Geometry check sheet. Reference: the model listing, model coordinates, mm. A direction names the side the tool comes from. Give positions to 0.01 mm unless a question says otherwise; leave off trailing zeros. Write each loop counter-clockwise with the first axis right and the second up, starting at its lowest first coordinate (ties: lowest second). Pieces come first, ordered by that corner, then holes.
(1) Tool access check on faces 4 (the flat face through (0, -1.588, -118)), 5 (the cylindrical face through (0.488, -0.805, -185.804)). Record the directions out of +Z, -Z, +X, -X, +Y, -Y that give a thin tool (end or side, any length) a straight path to the whole face; none if there is none.
(2) Cross-section at C-C (z = -180). Record the boundary of the cut face in (x, y).
(3) Cross-section at A-A (y = -9). Record the boundary of the cut face in (x, z).
(4) Cross-section at B-B (z = -7). Record the boundary of the cut face in (x, y).
(5) Mould release check, pull along Z, two halves, no side actions. Record for faces 1 (the flat face through (1, -1, 20)), 2 (the flat face through (-5.016, -7, -118)), 3 (the cylindrical face through (0.29, -0.8, 5.77)): +Z half, -Z half, draft (parallel to the pull), parting line (faces both ways), or undercut.
(6) Thickness scan on line 1 along X through (y, z) = (-5, -4); line 2 along X through (y, z) = (-0.5, -188); line 3 along Y through (x, z) = (-2, -82). Record the ranges inside material, lowest first.
(7) Depth check by flat-ended pin: P1, Ø5, axis at x = -2, z = -65.5, coming from the -Y side. Enter the tip coordinate at first touch or a pass-through.
```python
from build123d import *

# Parameters (mm, degrees)
BOSS_EXTRUDE1_DEPTH      = 20
BOSS_EXTRUDE1_DEPTH_BACK = 260
M4_CLEARANCE_HOLE1_D     = 4.5
M4_CLEARANCE_HOLE2_D     = 4.5


with BuildPart() as part:
    # Sketch1 → Boss-Extrude1 (new body, two sides)
    with BuildSketch(Plane.XY) as boss_extrude1_sk:
        Polygon((-6.604, 0), (6.604, 0), (6.604, -12.7), (5.0165, -12.7), (5.0165, -1.5875), (-5.0165, -1.5875), (-5.0165, -12.7), (-6.604, -12.7), align=None)
    extrude(amount=BOSS_EXTRUDE1_DEPTH)
    extrude(boss_extrude1_sk.sketch, amount=-BOSS_EXTRUDE1_DEPTH_BACK)

    # M4 Clearance Hole1 (through all)
    with Locations(Plane(origin=(0, 0, 0), x_dir=(1, 0, 0), z_dir=(0, 1, 0))):
        with Locations((0, 7), (0, 248.64)):
            Hole(M4_CLEARANCE_HOLE1_D / 2)

    # M4 Clearance Hole2 (through all)
    with Locations(Plane(origin=(0, 0, 0), x_dir=(1, 0, 0), z_dir=(0, 1, 0))):
        with Locations((0, 108), (0, 128), (0, -8), (0, 188), (0, 168), (0, 68), (0, 48)):
            Hole(M4_CLEARANCE_HOLE2_D / 2)


solid = part.part
```
Reply:
1. face 4: +Z, -Z, -Y
1. face 5: +Y, -Y
2. outline: (-6.6, -12.7) - (-5.02, -12.7) - (-5.02, -1.59) - (5.02, -1.59) - (5.02, -12.7) - (6.6, -12.7) - (6.6, 0) - (-6.6, 0) - close
3. outline: (-6.6, -260) - (-5.02, -260) - (-5.02, 20) - (-6.6, 20) - close; (5.02, -260) - (6.6, -260) - (6.6, 20) - (5.02, 20) - close
4. outline: (-6.6, -12.7) - (-5.02, -12.7) - (-5.02, -1.59) - (-2.25, -1.59) - (-2.25, 0) - (-6.6, 0) - close; (2.25, -1.59) - (5.02, -1.59) - (5.02, -12.7) - (6.6, -12.7) - (6.6, 0) - (2.25, 0) - close
5. face 1: +Z half
5. face 2: draft
5. face 3: undercut
6. line 1: x = -6.6 to -5.02, 5.02 to 6.6
6. line 2: x = -6.6 to -2.25, 2.25 to 6.6
6. line 3: y = -1.59 to 0
7. P1: stops at y = -1.59
